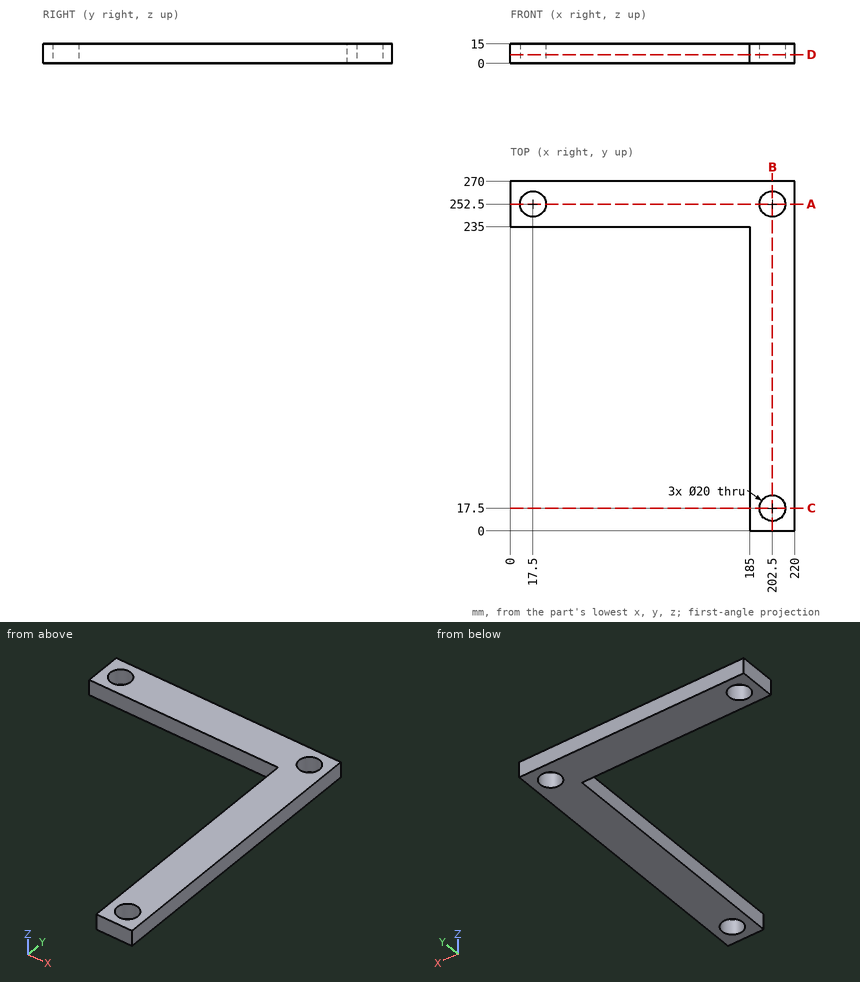
Check sheet for the drawn part. Datum: minimum x, y, z corner. Units: mm. Give positions to 0.01 mm unless a question says otherwise; leave off trailing zeros. Loops run counter-clockwise (first coordinate to the right, second up) from the corner with the lowest first, then second, coordinate; pieces in that order, holes last. Notation, with made-up numbers: M 23,15.25 L 76,15.25 A20 ccw 76,47.25 Z; hole C 51.25,72 d4. An arc over 180 degrees is marked long. Return JSON: item names as keys, results as strings.
1) Section check C-C, the plane y = 17.5. Enter the section's corners in (x, z).
Findings:
{"outline": "M 185,0 L 192.5,0 L 192.5,15 L 185,15 Z; M 212.5,0 L 220,0 L 220,15 L 212.5,15 Z"}
2) Section check B-B, the plane x = 202.5. Enter the section's corners in (y, z).
Findings:
{"outline": "M 0,0 L 7.5,0 L 7.5,15 L 0,15 Z; M 27.5,0 L 242.5,0 L 242.5,15 L 27.5,15 Z; M 262.5,0 L 270,0 L 270,15 L 262.5,15 Z"}
3) Gauge pin test, flat ends, axial feed: P1, Ø6, axis at y = 199, z = 8, coming from the -X side; P2, Ø1.5, axis at x = 193, y = 175.5, coming from the -Z side; P3, Ø1.5, axis at x = 92.5, z = 8, coming from the -Y side; P4, Ø12, axis at x = 202.5, y = 252.5, coming from the -Z side (1 decimal). Record the tip position at first contact, or that the pin passes through.
Findings:
{"P1": "stops at x = 185", "P2": "stops at z = 0", "P3": "stops at y = 235", "P4": "passes through"}
4) Section check D-D, the plane z = 6.75. Enter the section's corners in (x, y).
Findings:
{"outline": "M 0,235 L 185,235 L 185,0 L 220,0 L 220,270 L 0,270 Z; hole C 17.5,252.5 d20; hole C 202.5,17.5 d20; hole C 202.5,252.5 d20"}
5) Material ranges on L1, parallel to Y at x = 202.5, z = 4.75; L2, parallel to Y at x = 17.5, z = 8; L3, parallel to Y at x = 206.5, z = 3.5, recorded low to high. Write a range as [from, to].
Findings:
{"L1": "y = [0, 7.5], [27.5, 242.5], [262.5, 270]", "L2": "y = [235, 242.5], [262.5, 270]", "L3": "y = [0, 8.33], [26.67, 243.33], [261.67, 270]"}
6) Section check A-A, the plane y = 252.5. Enter the section's corners in (x, z).
Findings:
{"outline": "M 0,0 L 7.5,0 L 7.5,15 L 0,15 Z; M 27.5,0 L 192.5,0 L 192.5,15 L 27.5,15 Z; M 212.5,0 L 220,0 L 220,15 L 212.5,15 Z"}
